Design review of the part built by this model. Coordinates are the model's own, in mm. Round coordinates to 2 decimals unless told otherwise and drop trailing zeros. Write each loop counter-clockwise with the first axis right and the second up, starting at its lowest first coordinate (ties: lowest second). Pieces come first, ordered by that corner, then holes. Notation, with made-up numbers: M 39,-3 L 56,-3 A25 ccw 56,35 Z; hole C -19.75,74.25 d3. An arc over 180 degrees is marked long. One line per question, with ' | ' between items. Start each with the question number.
Item 1: For L1, parallel to Z at x = -18.5, y = 41.5; L2, parallel to X at y = 49, z = 16.75; L3, parallel to X at y = -35, z = 18, list the stretches that pass through material, from the lowest coordinate up.
Item 2: Draft analysis for pull direction Y (two halves, no side actions). For faces 1 (the face through (100, -1, 5)), 2 (the face through (-1, 100, 5)), 3 (the face through (-1, -100, 5)), 4 (the face through (-34.233, 54.591, 15.423)), state which applies: released by +Y, released by -Y, zero draft, split by the parting line, or undercut.
Item 3: Insertion check: pin 1 Ø1.5 at (y, z) = (-1.5, 12) entering from -X; pin 2 Ø5 at (x, z) = (-23.5, 17) entering from -Y. Each pin has a flat end and moves straight along its axis. Give the tip position at first contact, or say it passes through.
Item 4: Add section B-B, the plane y = 70. State the section outline as (x, z) points, and give its area (3 significant figures).
Item 5: Add section A-A, the plane x = -60. State the section outline as (y, z) points.
```python
from build123d import *

# Parameters (mm, degrees)
F0_W     = 200
F0_H     = 200
F1_DEPTH = 10
F2_R     = 5
F3_DEPTH = 12
F4_SIZE  = 1


with BuildPart() as f1:
    # F0 (on Top) → F1 (new body)
    with BuildSketch(Plane.XY):
        Rectangle(F0_W, F0_H)
    extrude(amount=F1_DEPTH)

    # F2 (on face) → F3 (join)
    with BuildSketch(Plane.XY.offset(10)):
        with BuildLine():
            Line((-60, -60), (-55, -60))
            ThreePointArc((-55, -60), (-55.4684610648, -57.8869086913), (-56.7860619516, -56.1697777844))
            Line((-56.7860619516, -56.1697777844), (-60, -60))
        make_face()
        with Locations((-39.0020143443, 53.0894473389)):
            Circle(F2_R)
        with BuildLine():
            ThreePointArc((7.9979856557, 53.0894473389), (10.1301034739, 48.9936871175), (14.7080863723, 48.390984235))
            Line((14.7080863723, 48.390984235), (12.9979856557, 53.0894473389))
            Line((12.9979856557, 53.0894473389), (7.9979856557, 53.0894473389))
        make_face()
        with BuildLine():
            Line((12.9979856557, 53.0894473389), (14.7080863723, 48.390984235))
            ThreePointArc((14.7080863723, 48.390984235), (17.0937458771, 50.2215651572), (17.9979856557, 53.0894473389))
            ThreePointArc((17.9979856557, 53.0894473389), (12.9979856557, 58.0894473389), (7.9979856557, 53.0894473389))
            Line((7.9979856557, 53.0894473389), (12.9979856557, 53.0894473389))
        make_face()
        with BuildLine():
            ThreePointArc((27.7048518187, 12.6826646451), (25.0848255164, 10.4842015412), (24.4909137702, 7.1159606529))
            Line((24.4909137702, 7.1159606529), (29.4149525353, 7.9842015412))
            Line((29.4149525353, 7.9842015412), (27.7048518187, 12.6826646451))
        make_face()
        with BuildLine():
            Line((29.4149525353, 7.9842015412), (24.4909137702, 7.1159606529))
            ThreePointArc((24.4909137702, 7.1159606529), (29.850731249, 3.0032280507), (34.4149525353, 7.9842015412))
            ThreePointArc((34.4149525353, 7.9842015412), (32.282834717, 12.0799617626), (27.7048518187, 12.6826646451))
            Line((27.7048518187, 12.6826646451), (29.4149525353, 7.9842015412))
        make_face()
        with BuildLine():
            ThreePointArc((-8.9925498322, 1.2119226122), (-16.603086639, 4.5606389529), (-16.784470779, -3.7520784976))
            Line((-16.784470779, -3.7520784976), (-13.9165885972, 0.3436817238))
            Line((-13.9165885972, 0.3436817238), (-8.9925498322, 1.2119226122))
        make_face()
        with BuildLine():
            Line((-13.9165885972, 0.3436817238), (-16.784470779, -3.7520784976))
            ThreePointArc((-16.784470779, -3.7520784976), (-11.6078455311, -4.091372442), (-8.9165885972, 0.3436817238))
            ThreePointArc((-8.9165885972, 0.3436817238), (-8.9356151068, 0.7794604376), (-8.9925498322, 1.2119226122))
            Line((-8.9925498322, 1.2119226122), (-13.9165885972, 0.3436817238))
        make_face()
        with BuildLine():
            ThreePointArc((-33.9917638695, -28.3266398263), (-40.8264127527, -29.3785929027), (-40.0735840997, -36.2526222633))
            Line((-40.0735840997, -36.2526222633), (-36.8596460513, -32.4224000477))
            Line((-36.8596460513, -32.4224000477), (-33.9917638695, -28.3266398263))
        make_face()
        with BuildLine():
            Line((-36.8596460513, -32.4224000477), (-40.0735840997, -36.2526222633))
            ThreePointArc((-40.0735840997, -36.2526222633), (-34.7465547426, -36.9539389829), (-31.8596460513, -32.4224000477))
            ThreePointArc((-31.8596460513, -32.4224000477), (-32.4245918854, -30.1136569815), (-33.9917638695, -28.3266398263))
            Line((-33.9917638695, -28.3266398263), (-36.8596460513, -32.4224000477))
        make_face()
        with BuildLine():
            ThreePointArc((-56.7860619516, -56.1697777844), (-64.5315389352, -62.1130913087), (-55, -60))
            Line((-55, -60), (-60, -60))
            Line((-60, -60), (-56.7860619516, -56.1697777844))
        make_face()
    extrude(amount=F3_DEPTH)

    # F4
    f4_edges = [f1.edges().sort_by_distance(p)[0] for p in [
        (-63.213938, -63.830222, 22),
        (-33.645708, -28.592178, 22),
        (-11.048706, 4.439442, 22),
        (11.287885, 57.78791, 22),
        (-44.002014, 53.089447, 22),
    ]]
    chamfer(f4_edges, length=F4_SIZE)


solid = f1.part
```
Computed values:
1) L1: z = 0 to 10 | L2: x = -41.88 to -36.13, 10.12 to 15.87 | L3: x = -41.14 to -32.58
2) face 1: zero draft | face 2: released by +Y | face 3: released by -Y | face 4: undercut
3) pin 1: stops at x = -18.8 | pin 2: passes through
4) outline: M -100,0 L 100,0 L 100,10 L -100,10 Z | area: 2,000 mm^2
5) outline: M -100,0 L 100,0 L 100,10 L -55,10 L -55,21 L -56,22 L -64,22 L -65,21 L -65,10 L -100,10 Z
